Part model, mm, in its own coordinate system. A direction names the side the tool comes from. Coordinates: 2 decimals unless noted, no trailing zeros. Order: outer loops, then holes, each group sorted by start corner. A loop starts at its lowest first (then second) coordinate and runs counter-clockwise, first axis right, second up.
1) Wall check: L1, parallel to X at y = 29.5, z = 0; L2, parallel to X at y = 6, z = 0 (3 decimals); L3, parallel to Z at x = -0.5, y = 23. Give the ranges that are in metal, low to high.
2) Mould opens along Y. For faces 4 (the cylindrical face through (3.755, 33.986, 11.923)), 5 (the flat face through (0, 35, 0)), 6 (the flat face through (-10, 33, 5)) say: +Y half, -Y half, draft (parallel to the pull), parting line (faces both ways), or undercut.
3) Cut at B-B (x = 0). List the corners of the cut face in (y, z) (1 decimal).
4) Cut at A-A (y = 29). List the corners of the cut face in (x, z).
5) Cut at C-C (z = 0). List the corners of the cut face in (x, y) (1 decimal).
6) Tool access for faces 1 (the flat face through (0, 9, 0)), 2 (the flat face through (-8, 3, -10)), 3 (the cylindrical face through (-10.74, 18.55, -2.38)): list every direction of +Z, -Z, +X, -X, +Y, -Y with a clear straight run to the whole face (end or side of a thin tool).
7) Pin check, flat tips, straight feed: pin 1 Ø5 at (x, y) = (10, 9.5) entering from -Z; pin 2 Ø2 at (x, y) = (-13, 12) entering from -Z; pin 3 Ø5 at (y, z) = (16.5, -14) entering from -X. Stop position of each tip, or through.
```python
from build123d import *

# Parameters (mm, degrees)
SKETCH1_R           = 17.5
SKETCH1_R_2         = 16
BOSS_EXTRUDE1_DEPTH = 34
SKETCH2_R           = 17.5
BOSS_EXTRUDE2_DEPTH = 3
FILLET1_R           = 2
SKETCH3_R           = 11
BOSS_EXTRUDE3_DEPTH = 30
CUT_EXTRUDE1_DEPTH  = 35
SKETCH6_W           = 7.99098924
SKETCH6_H           = 6.392791393
BOSS_EXTRUDE4_DEPTH = 24
FILLET3_R           = 1.5
SKETCH8_R           = 12.5
BOSS_EXTRUDE5_DEPTH = 2


with BuildPart() as part:
    # Sketch1 → Boss-Extrude1 (new body)
    with BuildSketch(Plane(origin=(0, 0, 0), x_dir=(1, 0, 0), z_dir=(0, 1, 0))):
        with Locations(Location((0, 0, 0), (0, 0, 270))):
            Circle(SKETCH1_R)
        with Locations(Location((0, 0, 0), (0, 0, 270))):
            Circle(SKETCH1_R_2, mode=Mode.SUBTRACT)
    extrude(amount=BOSS_EXTRUDE1_DEPTH)

    # Sketch2 → Boss-Extrude2 (add)
    with BuildSketch(Plane(origin=(0, 0, 0), x_dir=(1, 0, 0), z_dir=(0, 1, 0))):
        with Locations(Location((0, 0, 0), (0, 0, 270))):
            Circle(SKETCH2_R)
    extrude(amount=BOSS_EXTRUDE2_DEPTH)

    # Fillet1
    # the kernel refuses this fillet: 2 mm, written as the material it takes off along each edge
    with BuildSketch(Plane(origin=(0, 34, 0), x_dir=(0, 0, 1), z_dir=(-1, 0, 0))) as fillet1_piece_1:
        with BuildLine():
            CenterArc((18, -1.936491673), FILLET1_R, 104.477512186, 75.522487814)
            Line((16, -1.936491673), (15.96, -1.936491673))
            Line((15.96, -1.936491673), (15.96, 0))
            Line((15.96, 0), (16, 0.04))
            ThreePointArc((16, 0.04), (16.75, 0.04), (17.49, 0.038729833))
            Line((17.49, 0.038729833), (17.5, 0))
        make_face()
    revolve(axis=Axis((0, 34, 0), (0, 1, 0)), mode=Mode.SUBTRACT)

    # Sketch3 → Boss-Extrude3 (add)
    with BuildSketch(Plane(origin=(0, 3, 0), x_dir=(1, 0, 0), z_dir=(0, 1, 0))):
        with Locations(Location((0, 0, 0), (0, 0, 270))):
            Circle(SKETCH3_R)
    extrude(amount=BOSS_EXTRUDE3_DEPTH)

    # Sketch5 → Cut-Extrude1 (cut)
    with BuildSketch(Plane(origin=(0, 33, 0), x_dir=(1, 0, 0), z_dir=(0, 1, 0))):
        with BuildLine():
            Line((-1.077438314, 1.385334501), (1.077438314, 1.385334501))
            ThreePointArc((1.077438314, 1.385334501), (0, -1.755), (-1.077438314, 1.385334501))
        make_face()
    extrude(amount=-CUT_EXTRUDE1_DEPTH, mode=Mode.SUBTRACT)

    # Sketch6 → Boss-Extrude4 (add)
    with BuildSketch(Plane(origin=(0, 33, 0), x_dir=(1, 0, 0), z_dir=(0, 1, 0))):
        with Locations((0.014035957, -0.788514839)):
            Rectangle(SKETCH6_W, SKETCH6_H)
    extrude(amount=-BOSS_EXTRUDE4_DEPTH)

    # Fillet3
    fillet3_edges = [part.edges().sort_by_distance(p)[0] for p in [
        (0, 3, -11),
    ]]
    fillet(fillet3_edges, radius=FILLET3_R)

    # Sketch8 → Boss-Extrude5 (add)
    with BuildSketch(Plane(origin=(0, 33, 0), x_dir=(1, 0, 0), z_dir=(0, 1, 0))):
        with Locations(Location((0, 0, 0), (0, 0, 270))):
            Circle(SKETCH8_R)
    extrude(amount=BOSS_EXTRUDE5_DEPTH)


solid = part.part
```
Geometry check:
1. L1: x = -17.5 to -16, -11 to 11, 16 to 17.5
1. L2: x = -17.5 to -16, -11 to -1.755, 1.755 to 11, 16 to 17.5
1. L3: z = -17.49 to -15.99, -10.99 to 10.99, 15.99 to 17.49
2. face 4: draft
2. face 5: +Y half
2. face 6: undercut
3. outline: (0, -17.5) - (34, -17.5) arc R2 ccw to (32.1, -16) - (3, -16) - (3, -12.5) arc R1.5 cw to (4.5, -11) - (33, -11) - (33, -12.5) - (35, -12.5) - (35, 12.5) - (33, 12.5) - (33, 11) - (4.5, 11) arc R1.5 cw to (3, 12.5) - (3, 16) - (32.1, 16) arc R2 ccw to (34, 17.5) - (0, 17.5) - (0, 1.8) - (9, 1.8) - (9, -1.4) - (0, -1.4) - close
4. outline: circle Ø35 at (0, 0); circle Ø22 at (0, 0); hole circle Ø32 at (0, 0)
5. outline: (-17.5, 0) - (-1.8, 0) - (-1.8, 9) - (1.8, 9) - (1.8, 0) - (17.5, 0) - (17.5, 34) arc R2 ccw to (16, 32.1) - (16, 3) - (12.5, 3) arc R1.5 cw to (11, 4.5) - (11, 33) - (12.5, 33) - (12.5, 35) - (-12.5, 35) - (-12.5, 33) - (-11, 33) - (-11, 4.5) arc R1.5 cw to (-12.5, 3) - (-16, 3) - (-16, 32.1) arc R2 ccw to (-17.5, 34) - close
6. face 1: -Y
6. face 2: +Y
6. face 3: none
7. pin 1: stops at z = -15.81
7. pin 2: stops at z = -12.74
7. pin 3: stops at x = -13.19
